Check sheet for the modelled part. Datum: model origin and axes. Units: mm. Face numbers are marked on the shaded views. A direction names the side the tool comes from. Round coordinates to 2 decimals unless told otherwise and drop trailing zeros. Write each loop counter-clockwise with the first axis right and the second up, starting at its lowest first coordinate (ties: lowest second). Pieces come first, ordered by that corner, then holes. Notation, with made-up numbers: (65, -18) -> (78, -18) arc R16 ccw to (78, -2) -> close; hole circle Ø10 at (28, -18). An arc over 180 degrees is marked (long way). Use one line per item in the form item = value. Start each with the question number.
```python
from build123d import *

# Parameters (mm, degrees)
F0_W     = 50
F0_H     = 50
F1_DEPTH = 50
F2_T     = -5
F3_R     = 9
F4_SIZE  = 4.99999


# Not quite as in the source:
# - a fillet or chamfer is up to 0.001 mm smaller than in the source, because OpenCascade refuses the exact size


with BuildPart() as f1:
    # F0 (on Top) → F1 (new body)
    with BuildSketch(Plane.XY):
        Rectangle(F0_W, F0_H)
    extrude(amount=F1_DEPTH)

    # F2
    f2_openings = [f1.faces().sort_by_distance(p)[0] for p in [
        (0, 0, 50),
    ]]
    offset(amount=F2_T, openings=f2_openings)

    # F3
    f3_edges = [f1.edges().sort_by_distance(p)[0] for p in [
        (-25, 25, 25),
        (-25, -25, 25),
        (25, -25, 25),
        (25, 25, 25),
        (20, -20, 27.5),
        (-20, -20, 27.5),
        (-20, 20, 27.5),
        (20, 20, 27.5),
    ]]
    fillet(f3_edges, radius=F3_R)

    # F4 (size 5 in the source; OpenCascade refuses exactly that, so slightly less here)
    f4_edges = [f1.edges().sort_by_distance(p)[0] for p in [
        (25, 0, 0),
        (25, -16, 25),
        (25, 16, 25),
        (25, 0, 50),
        (0, 25, 0),
        (16, 25, 25),
        (-16, 25, 25),
        (0, 25, 50),
        (-25, 0, 0),
        (-25, 16, 25),
        (-25, -16, 25),
        (-25, 0, 50),
        (0, -25, 0),
        (-16, -25, 25),
        (16, -25, 25),
        (0, -25, 50),
    ]]
    chamfer(f4_edges, length=F4_SIZE)


solid = f1.part
```
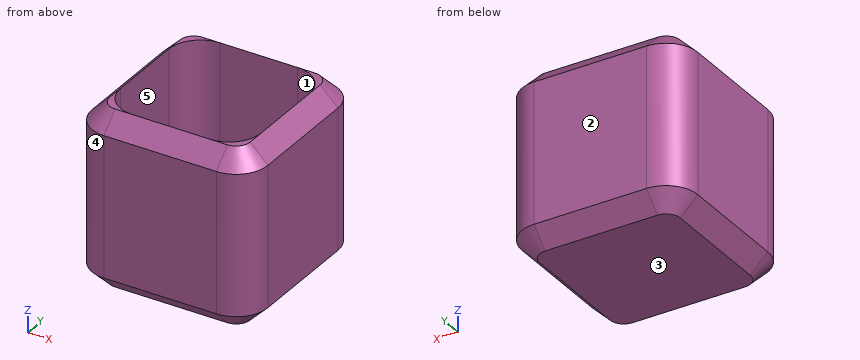
1. Sectioned sample at D-D (z = 46). Enter the section's corners in (x, y).
2. Depth check by flat-ended pin: pin 1 (4 mm diameter, centred on x = 7, y = -4, fed in from +Z). Enter the tip coordinate at first touch or a pass-through.
3. Tool access check on the marked faces 4 and 5. Record the directions out of +Z, -Z, +X, -X, +Y, -Y that give a thin tool (end or side, any length) a straight path to the whole face; none if there is none.
4. Scan lines: probe 1 along Y at (x, z) = (-4, 44.5); probe 2 along Z at (x, y) = (11, 6.5). Record each from-to range of solid material in increasing order.
5. Sectioned sample at A-A (z = 35). Enter the section's corners in (x, y).
6. Mould release check, pull along Y, two halves, no side actions. Record for the marked faces 1, 2 and 3: +Y half, -Y half, draft (parallel to the pull), parting line (faces both ways), or undercut.
Returned:
q1.outline = (-24, -16) arc R8 ccw to (-16, -24) -> (16, -24) arc R8 ccw to (24, -16) -> (24, 16) arc R8 ccw to (16, 24) -> (-16, 24) arc R8 ccw to (-24, 16) -> close; hole (-20, -11) arc R9 ccw to (-11, -20) -> (11, -20) arc R9 ccw to (20, -11) -> (20, 11) arc R9 ccw to (11, 20) -> (-11, 20) arc R9 ccw to (-20, 11) -> close
q2.pin_1 = 5
q3.face_4 = +Z, -Z, -X, -Y
q3.face_5 = +Z
q4.probe_1 = -25 to -20, 20 to 25
q4.probe_2 = 0 to 5
q5.outline = (-25, -16) arc R9 ccw to (-16, -25) -> (16, -25) arc R9 ccw to (25, -16) -> (25, 16) arc R9 ccw to (16, 25) -> (-16, 25) arc R9 ccw to (-25, 16) -> close; hole (-20, -11) arc R9 ccw to (-11, -20) -> (11, -20) arc R9 ccw to (20, -11) -> (20, 11) arc R9 ccw to (11, 20) -> (-11, 20) arc R9 ccw to (-20, 11) -> close
q6.face_1 = undercut
q6.face_2 = +Y half
q6.face_3 = draft
